Can you work these out from the model? Positions are in its coordinate system, mm. Face numbers are marked on the shaded views. A direction names the side the tool comes from. Coordinates: 2 decimals unless noted, no trailing zeros. Order: outer loops, then holes, each group sorted by start corner. A loop starts at its lowest first (then second) coordinate and runs counter-clockwise, first axis right, second up.
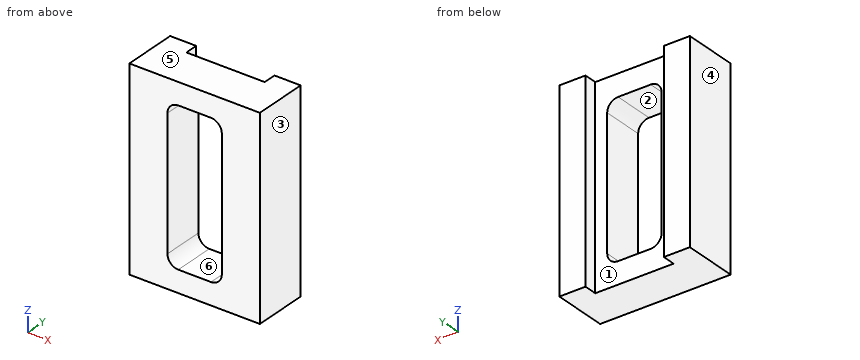
```python
from build123d import *

# Parameters (mm, degrees)
F0_W     = 60
F0_H     = 90
F0_W_2   = 25
F0_H_2   = 70
F1_DEPTH = 12.5
F2_W     = 36
F2_H     = 6
F3_DEPTH = 90.001
F4_R     = 5


with BuildPart() as f1:
    # F0 (on Front) → F1 (new body, symmetric)
    with BuildSketch(Plane.XZ):
        Rectangle(F0_W, F0_H)
        Rectangle(F0_W_2, F0_H_2, mode=Mode.SUBTRACT)
    extrude(amount=F1_DEPTH, both=True)

    # F2 (on face) → F3 (cut, through all)
    with BuildSketch(Plane.XY.offset(45)):
        with Locations((0, 9.5)):
            Rectangle(F2_W, F2_H)
    extrude(amount=-F3_DEPTH, mode=Mode.SUBTRACT)

    # F4
    f4_edges = [f1.edges().sort_by_distance(p)[0] for p in [
        (-12.5, -3, 35),
        (12.5, -3, 35),
        (12.5, -3, -35),
        (-12.5, -3, -35),
    ]]
    fillet(f4_edges, radius=F4_R)


solid = f1.part
```
1. Imagine slicing it at B-B on y = -5. Please give me the cut outline in (x, z).
Completed:
outline: (-30, -45) - (30, -45) - (30, 45) - (-30, 45) - close; hole (-12.5, -30) arc R5 ccw to (-7.5, -35) - (7.5, -35) arc R5 ccw to (12.5, -30) - (12.5, 30) arc R5 ccw to (7.5, 35) - (-7.5, 35) arc R5 ccw to (-12.5, 30) - close
2. On a 3-axis mill with a long thin cutter (end or side, diameter ignored), from which of +Z, -Z, +X, -X, +Y, -Y can I reach the whole of each face in a straight line? I mean the marked faces 1, 2 and 3. Say none if no direction works.
Completed:
face 1: +Z, -Z, +Y
face 2: +Y, -Y
face 3: +Z, -Z, +X, +Y, -Y
3. Imagine slicing it at C-C on x = -3. Please give me the cut outline in (y, z), then the cut area to 3 significant figures.
Completed:
outline: (-12.5, -45) - (6.5, -45) - (6.5, -35) - (-12.5, -35) - close; (-12.5, 35) - (6.5, 35) - (6.5, 45) - (-12.5, 45) - close
area: 380 mm2
4. Thinking about a two-plate mould opening in Z: for the marked faces 4, 5 and 6, which applies, pulls with the +Z half, pulls with the -Z half, needs draft (parallel to the pull), parting line crosses it, or undercut?
Completed:
face 4: needs draft
face 5: pulls with the +Z half
face 6: undercut
5. Please list where these lines run through material, in increasing order: probe 1 along X at (y, z) = (7.25, 8); probe 2 along X at (y, z) = (2.5, 0.5); probe 3 along Z at (x, y) = (-6.5, 4).
Completed:
probe 1: x = -30 to -18, 18 to 30
probe 2: x = -30 to -12.5, 12.5 to 30
probe 3: z = -45 to -35, 35 to 45
6. Imagine slicing it at A-A on z = -33. Please give me the cut outline in (x, y), then the cut area to 3 significant figures.
Completed:
outline: (-30, -12.5) - (-11.5, -12.5) - (-11.5, 6.5) - (-18, 6.5) - (-18, 12.5) - (-30, 12.5) - close; (11.5, -12.5) - (30, -12.5) - (30, 12.5) - (18, 12.5) - (18, 6.5) - (11.5, 6.5) - close
area: 847 mm2
7. Imagine slicing it at D-D on y = 10.5. Please give me the cut outline in (x, z), then the cut area to 3 significant figures.
Completed:
outline: (-30, -45) - (-18, -45) - (-18, 45) - (-30, 45) - close; (18, -45) - (30, -45) - (30, 45) - (18, 45) - close
area: 2,160 mm2
